Verification items for the finished model (mm, model axes). Face numbers are marked on the shaded views. A direction names the side the tool comes from. Round coordinates to 2 decimals unless told otherwise and drop trailing zeros. Write each loop counter-clockwise with the first axis right and the second up, starting at its lowest first coordinate (ties: lowest second). Pieces come first, ordered by that corner, then holes. Notation, with made-up numbers: M 4.5,16 L 53.5,16 A12 cw 53.5,39 Z; hole C 13.25,56 d7. An arc over 180 degrees is marked long. One line per item, written item: value. Start each with the question number.
Item 1: Gauge pin test, flat ends, axial feed: pin 1 (3 mm diameter, centred on x = 4.5, z = 11.5, fed in from +Y); pin 2 (1 mm diameter, centred on y = -14.5, z = 7.5, fed in from -X); pin 3 (12 mm diameter, centred on y = -15.5, z = 0, fed in from -X); pin 4 (1.5 mm diameter, centred on x = 4, z = 6.5, fed in from -Y). Record the tip position at first contact, or that the pin passes through.
Item 2: Section check A-A, the plane y = -18. Record the cut outline in (x, z).
Item 3: Tool access check on the marked faces 1, 2 and 3. Record the directions out of +Z, -Z, +X, -X, +Y, -Y that give a thin tool (end or side, any length) a straight path to the whole face; none if there is none.
Item 4: Thickness scan on probe 1 along Z at (x, y) = (0.9, -12.5); probe 2 along Z at (x, y) = (3.85, 9.5); probe 3 along Y at (x, z) = (0.5, -17). Record the ranges inside material, lowest first. Write a range as from..to.
Item 5: Draft check along Z on the marked faces 4, 5 and 6. Enter one of: +Z half, -Z half, draft (parallel to the pull), parting line (faces both ways), or undercut.
Item 6: Section check C-C, the plane z = 14.5. Record the cut outline in (x, y), then the cut area to 3 significant figures.
Item 7: Section check B-B, the plane y = 14.5. Record the cut outline in (x, z).
from build123d import *

# Parameters (mm, degrees)
SKETCH_R           = 10.375
PAD_DEPTH          = 5
POCKET_DEPTH       = 2
PAD001_DEPTH       = 10
PAD001_DEPTH_BACK  = 1
POLARPATTERN_COUNT = 20


with BuildPart() as part:
    # Sketch → Pad (new body)
    with BuildSketch(Plane.YZ):
        Circle(SKETCH_R)
    extrude(amount=PAD_DEPTH)

    # Sketch001 (on Face3 of Pad) → Pocket (cut)
    with BuildSketch(Plane.YZ.offset(5)):
        Polygon((2.165064, 1.25), (0, 2.5), (-2.165064, 1.25), (-2.165064, -1.25), (0, -2.5), (2.165064, -1.25), align=None)
    extrude(amount=-POCKET_DEPTH, mode=Mode.SUBTRACT)

    # Sketch002 (on DatumPlane) → Pad001 (join, two sides)
    with BuildSketch(Plane.ZX.offset(10.375)) as pad001_sk:
        Polygon((0.8, 0), (-0.3, 5), (-0.8, 5), (0.3, 0), align=None)
    pad001 = extrude(amount=PAD001_DEPTH) + extrude(pad001_sk.sketch, amount=-PAD001_DEPTH_BACK)

    # PolarPattern: Pad001 ×20 about axis
    polarpattern_axis = Axis((0, 0, 0), (1, 0, 0))
    for i in range(1, POLARPATTERN_COUNT):
        add(pad001.rotate(polarpattern_axis, i * 360 / POLARPATTERN_COUNT))


solid = part.part
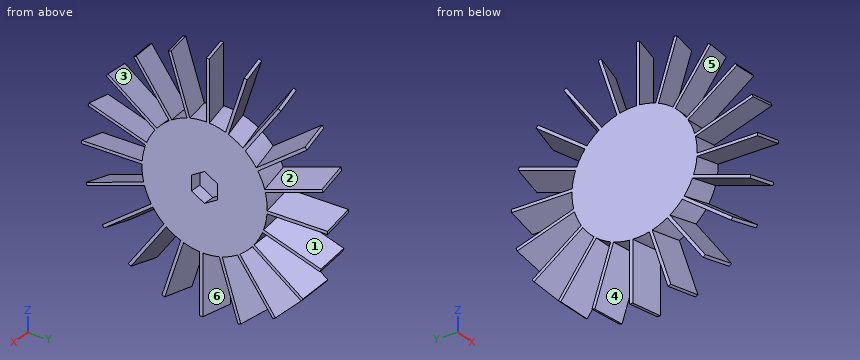
Response values:
1. pin 1: stops at y = 16.95
1. pin 2: passes through
1. pin 3: stops at x = 0
1. pin 4: stops at y = -19.4
2. outline: M 0,-6.69 L 5,-5.53 L 5,-5.01 L 0,-6.16 Z; M 0,-0.8 L 5,0.3 L 5,0.8 L 0,-0.3 Z; M 0,5.01 L 5,6.16 L 5,6.69 L 0,5.53 Z
3. face 1: +X, +Y
3. face 2: +X
3. face 3: -X
4. probe 1: z = -9.83..-9.21, -4.69..-4.17, -0.6..-0.1, 3.43..3.95, 8.34..8.96
4. probe 2: z = -14.01..-13.16, -7.58..-6.96, -4.17..4.17, 6.23..6.84, 12.15..13
4. probe 3: y = -5.32..-4.8, 0.19..0.69, 5.72..6.25
5. face 4: -Z half
5. face 5: undercut
5. face 6: draft
6. outline: M 0,-11.52 L 5,-10.16 L 5,-9.55 L 0,-10.91 Z; M 0,-5.55 L 5,-4.4 L 5,-3.87 L 0,-5.03 Z; M 0,-0.8 L 5,0.3 L 5,0.8 L 0,-0.3 Z; M 0,3.87 L 5,5.03 L 5,5.55 L 0,4.4 Z; M 0,9.55 L 5,10.91 L 5,11.52 L 0,10.16 Z
6. area: 13.9 mm2
7. outline: M 0,-10.16 L 5,-11.52 L 5,-10.91 L 0,-9.55 Z; M 0,-4.4 L 5,-5.55 L 5,-5.03 L 0,-3.87 Z; M 0,0.3 L 5,-0.8 L 5,-0.3 L 0,0.8 Z; M 0,5.03 L 5,3.87 L 5,4.4 L 0,5.55 Z; M 0,10.91 L 5,9.55 L 5,10.16 L 0,11.52 Z
